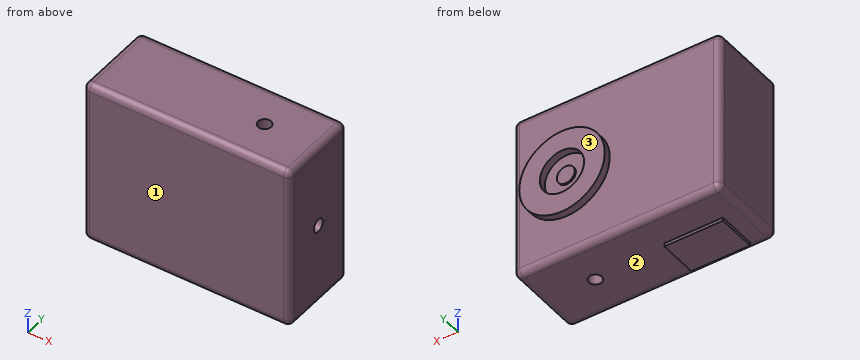
```python
from build123d import *

# Parameters (mm, degrees)
SKETCH1_W           = 63.5
SKETCH1_H           = 50.8
BOSS_EXTRUDE1_DEPTH = 25.2
SKETCH2_R           = 13.1445
SKETCH2_R_2         = 6.7945
BOSS_EXTRUDE2_DEPTH = 2.2
SKETCH3_R           = 2
CUT_EXTRUDE1_DEPTH  = 5.5
SKETCH4_R           = 2
CUT_EXTRUDE2_DEPTH  = 5.5
CUT_EXTRUDE3_START  = -5.5
SKETCH5_R           = 2
CUT_EXTRUDE3_DEPTH  = 5.5
FILLET1_R           = 2
SKETCH6_W           = 18
SKETCH6_H           = 12
BOSS_EXTRUDE3_DEPTH = 1
SKETCH7_R           = 2.75
BOSS_EXTRUDE4_DEPTH = 0.5


with BuildPart() as part:
    # Sketch1 → Boss-Extrude1 (new body)
    with BuildSketch(Plane(origin=(0, 0, 0), x_dir=(1, 0, 0), z_dir=(0, 1, 0))):
        Rectangle(SKETCH1_W, SKETCH1_H)
    extrude(amount=BOSS_EXTRUDE1_DEPTH)

    # Sketch2 → Boss-Extrude2 (add)
    with BuildSketch(Plane(origin=(0, 25.2, 0), x_dir=(1, 0, 0), z_dir=(0, 1, 0))):
        with Locations(Location((15.25, 0, 0), (0, 0, 90))):
            Circle(SKETCH2_R)
        with Locations(Location((15.25, 0, 0), (0, 0, 270))):
            Circle(SKETCH2_R_2, mode=Mode.SUBTRACT)
    extrude(amount=BOSS_EXTRUDE2_DEPTH)

    # Sketch3 → Cut-Extrude1 (cut)
    with BuildSketch(Plane.XY.offset(25.4)):
        with Locations((15.25, 12.6)):
            Circle(SKETCH3_R)
    extrude(amount=-CUT_EXTRUDE1_DEPTH, mode=Mode.SUBTRACT)

    # Sketch4 → Cut-Extrude2 (cut)
    with BuildSketch(Plane(origin=(31.75, 0, 0), x_dir=(0, 0, -1), z_dir=(1, 0, 0))):
        with Locations((0, 12.6)):
            Circle(SKETCH4_R)
    extrude(amount=-CUT_EXTRUDE2_DEPTH, mode=Mode.SUBTRACT)

    # Sketch5 → Cut-Extrude3 (cut)
    with BuildSketch(Plane(origin=(0, 0, -25.4), x_dir=(-1, 0, 0), z_dir=(0, 0, -1)).offset(CUT_EXTRUDE3_START)):
        with Locations(Location((-15.25, 12.6, 0), (0, 0, 180))):
            Circle(SKETCH5_R)
    extrude(amount=CUT_EXTRUDE3_DEPTH, mode=Mode.SUBTRACT)

    # Fillet1
    fillet1_edges = [part.edges().sort_by_distance(p)[0] for p in [
        (-31.75, 25.2, 0),
        (0, 25.2, 25.4),
        (31.75, 25.2, 0),
        (0, 0, 25.4),
        (-31.75, 0, 0),
        (0, 0, -25.4),
        (31.75, 0, 0),
        (0, 25.2, -25.4),
        (31.75, 12.6, 25.4),
        (-31.75, 12.6, 25.4),
        (-31.75, 12.6, -25.4),
        (31.75, 12.6, -25.4),
    ]]
    fillet(fillet1_edges, radius=FILLET1_R)

    # Sketch6 → Boss-Extrude3 (add)
    with BuildSketch(Plane(origin=(0, 0, -25.4), x_dir=(-1, 0, 0), z_dir=(0, 0, -1))):
        with Locations((16.25, 8.5)):
            Rectangle(SKETCH6_W, SKETCH6_H)
    extrude(amount=BOSS_EXTRUDE3_DEPTH)

    # Sketch7 → Boss-Extrude4 (add)
    with BuildSketch(Plane(origin=(0, 25.2, 0), x_dir=(1, 0, 0), z_dir=(0, 1, 0))):
        with Locations(Location((15.25, 0, 0), (0, 0, 90))):
            Circle(SKETCH7_R)
    extrude(amount=BOSS_EXTRUDE4_DEPTH)


solid = part.part
```
Check sheet for the modelled part. Datum: model origin and axes. Units: mm. Face numbers are marked on the shaded views. Coordinates: 2 decimals unless noted, no trailing zeros. Write each loop counter-clockwise with the first axis right and the second up, starting at its lowest first coordinate (ties: lowest second). Pieces come first, ordered by that corner, then holes. Notation, with made-up numbers: (16.25, 49.25) - (44.25, 49.25) arc R17 cw to (44.25, 66.25) - close; hole circle Ø4 at (85.25, 55.5). An arc over 180 degrees is marked (long way). One line per question, with ' | ' between items.
Item 1: Sectioned sample at D-D on z = 16. Record the boundary of the cut face in (x, y).
Determined:
outline: (-31.75, 2) arc R2 ccw to (-29.75, 0) - (29.75, 0) arc R2 ccw to (31.75, 2) - (31.75, 23.2) arc R2 ccw to (29.75, 25.2) - (-29.75, 25.2) arc R2 ccw to (-31.75, 23.2) - close
Item 2: Thickness scan on line 1 (Y direction, x = 15, z = 22); line 2 (X direction, y = 12.6, z = -23.65); line 3 (Y direction, x = 27.9, z = 0). Record the ranges inside material, lowest first. Write a range as [from, to].
Determined:
line 1: y = [0, 10.62], [14.58, 25.2] | line 2: x = [-31.73, 13.25], [17.25, 31.73] | line 3: y = [0, 10.6], [14.6, 27.4]
Item 3: Sectioned sample at C-C on y = 12.6. Record the boundary of the cut face in (x, z).
Determined:
outline: (-31.75, -23.4) arc R2 ccw to (-29.75, -25.4) - (-25.25, -25.4) - (-25.25, -26.4) - (-7.25, -26.4) - (-7.25, -25.4) - (13.25, -25.4) - (13.25, -19.9) - (17.25, -19.9) - (17.25, -25.4) - (29.75, -25.4) arc R2 ccw to (31.75, -23.4) - (31.75, -2) - (26.25, -2) - (26.25, 2) - (31.75, 2) - (31.75, 23.4) arc R2 ccw to (29.75, 25.4) - (17.25, 25.4) - (17.25, 19.9) - (13.25, 19.9) - (13.25, 25.4) - (-29.75, 25.4) arc R2 ccw to (-31.75, 23.4) - close
Item 4: Sectioned sample at A-A on x = -13.5. Record the boundary of the cut face in (y, z).
Determined:
outline: (0, -23.4) arc R2 ccw to (2, -25.4) - (2.5, -25.4) - (2.5, -26.4) - (14.5, -26.4) - (14.5, -25.4) - (23.2, -25.4) arc R2 ccw to (25.2, -23.4) - (25.2, 23.4) arc R2 ccw to (23.2, 25.4) - (2, 25.4) arc R2 ccw to (0, 23.4) - close
Item 5: Sectioned sample at B-B on z = 0. Record the boundary of the cut face in (x, y).
Determined:
outline: (-31.75, 2) arc R2 ccw to (-29.75, 0) - (29.75, 0) arc R2 ccw to (31.75, 2) - (31.75, 10.6) - (26.25, 10.6) - (26.25, 14.6) - (31.75, 14.6) - (31.75, 23.2) arc R2 ccw to (29.75, 25.2) - (28.39, 25.2) - (28.39, 27.4) - (22.04, 27.4) - (22.04, 25.2) - (18, 25.2) - (18, 25.7) - (12.5, 25.7) - (12.5, 25.2) - (8.46, 25.2) - (8.46, 27.4) - (2.11, 27.4) - (2.11, 25.2) - (-29.75, 25.2) arc R2 ccw to (-31.75, 23.2) - close
Item 6: Gauge pin test, flat ends, axial feed: P1, Ø8, axis at x = 15.25, z = 0, coming from the +Y side; P2, Ø3, axis at x = 15.25, y = 12.6, coming from the +Z side; P3, Ø4, axis at x = -15.5, y = 22, coming from the -Z side. Record the tip position at first contact, or that the pin passes through.
Determined:
P1: stops at y = 25.7 | P2: stops at z = 19.9 | P3: stops at z = -25.4
Item 7: Mould release check, pull along Y, two halves, no side actions. Record for the marked faces 1, 2 and 3: pulls with the +Y half, pulls with the -Y half, needs draft (parallel to the pull), parting line crosses it, or undercut.
Determined:
face 1: pulls with the -Y half | face 2: needs draft | face 3: pulls with the +Y half
